Geometry: final body of the model. Coordinates: model frame, mm. Round coordinates to 2 decimals unless told otherwise and drop trailing zeros. Loops run counter-clockwise (first coordinate to the right, second up) from the corner with the lowest first, then second, coordinate; pieces in that order, holes last. Notation, with made-up numbers: (19.25, 87.5) - (58.25, 87.5) arc R19 ccw to (58.25, 117.5) - close; hole circle Ø9 at (20, -30). An arc over 180 degrees is marked (long way). Return JSON: item names as keys, results as strings. Group by question number.
1. Material intervals for probe 1 along Y at (x, z) = (67, 4) (3 decimals); probe 2 along Y at (x, z) = (3.5, 5.25); probe 3 along Y at (x, z) = (52.5, 2.25) (3 decimals), sorted ascending.
2. First-contact query: pin 1 Ø3 at (y, z) = (34.5, 3) entering from -X; pin 2 Ø1.9 at (x, z) = (55.5, 4) entering from +Y; pin 3 Ø1.5 at (x, z) = (-50, 5.5) entering from -Y. Flat tips, straight axial feed; report the tip coordinate or a pass-through.
3. Section A-A on z = 3. Return loops of the section in (x, y) (3 decimals), and give its area (3 significant figures).
4. Section D-D on x = 13. Return loops of the section in (y, z).
5. Section B-B on x = -61. Return loops of the section in (y, z) (3 decimals).
6. Section C-C on y = 0. Return loops of the section in (x, z).
from build123d import *

# Parameters (mm, degrees)
SKETCH1_R           = 73.66
BOSS_EXTRUDE1_DEPTH = 6.35
CUT_EXTRUDE1_DEPTH  = 7.35


with BuildPart() as part:
    # Sketch1 → Boss-Extrude1 (new body)
    with BuildSketch(Plane.XY):
        Circle(SKETCH1_R)
    extrude(amount=BOSS_EXTRUDE1_DEPTH)

    # Sketch2 → Cut-Extrude1 (cut, through all)
    with BuildSketch(Plane(origin=(0, 0, 0), x_dir=(-1, 0, 0), z_dir=(0, 0, -1))):
        Polygon((-48.26, 0), (-48.26, 3.175), (-76.2, 3.175), (-76.2, -3.175), (-48.26, -3.175), align=None)
        Polygon((48.26, -3.175), (48.26, 0), (48.26, 3.175), (76.2, 3.175), (76.2, -3.175), align=None)
    extrude(amount=-CUT_EXTRUDE1_DEPTH, mode=Mode.SUBTRACT)


solid = part.part
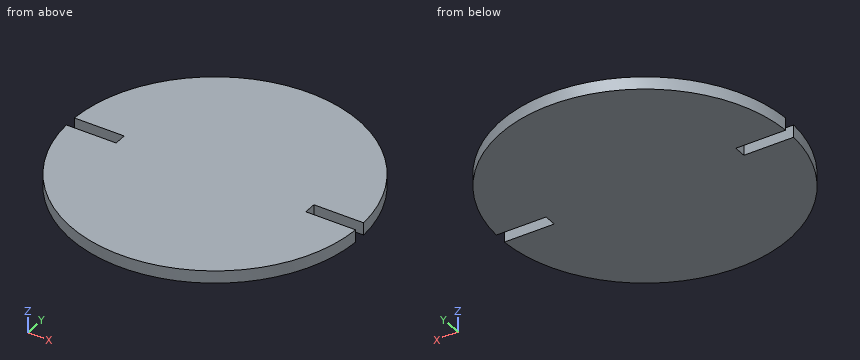
Taken from the geometry:
{
 "1": {"probe 1": "-30.607 to -3.175, 3.175 to 30.607", "probe 2": "-73.58 to 73.58", "probe 3": "-51.668 to -3.175, 3.175 to 51.668"},
 "2": {"pin 1": "x = -65.85", "pin 2": "y = 49.5", "pin 3": "y = -54.77"},
 "3": {"outline": "(-73.592, -3.175) arc R73.66 ccw to (73.592, -3.175) - (48.26, -3.175) - (48.26, 3.175) - (73.592, 3.175) arc R73.66 ccw to (-73.592, 3.175) - (-48.26, 3.175) - (-48.26, -3.175) - close", "area": "16,700 mm2"},
 "4": {"outline": "(-72.5, 0) - (72.5, 0) - (72.5, 6.35) - (-72.5, 6.35) - close"},
 "5": {"outline": "(-41.289, 0) - (-3.175, 0) - (-3.175, 6.35) - (-41.289, 6.35) - close; (3.175, 0) - (41.289, 0) - (41.289, 6.35) - (3.175, 6.35) - close"},
 "6": {"outline": "(-48.26, 0) - (48.26, 0) - (48.26, 6.35) - (-48.26, 6.35) - close"}
}
